Autodesk Inventor part; units mm, degrees
ref_plane "Work Plane1" through (-21.9731, -18.5883, -14.2) normal (0, 0, -1) x (0, 1, 0)
ref_plane "YZ Plane" through (0, 0, 0) normal (1, 0, 0) x (0, 1, 0)
ref_plane "XZ Plane" through (0, 0, 0) normal (0, 1, 0) x (-1, 0, 0)
sketch "Sketch1" plane through (0, 0, 0) normal (0, 0, 1) x (1, 0, 0)
  line L0 (-11, 18.9) -> (-11, 18.25)
  line L1 (-11, 18.25) -> (-20.7, 18.25)
  line L2 (-20.7, 18.25) -> (-20.7, -18.25)
  line L3 (-11, -18.25) -> (-20.7, -18.25)
  line L4 (-11, -18.25) -> (-11, -18.9)
  line L5 (0, -18.9) -> (-11, -18.9)
  line L6 (0, -18.25) -> (0, -18.9)
  line L7 (9.7, -18.25) -> (0, -18.25)
  line L8 (9.7, 18.25) -> (9.7, -18.25)
  line L9 (9.7, 18.25) -> (0, 18.25)
  line L10 (0, 18.9) -> (0, 18.25)
  line L11 (0, 18.9) -> (-11, 18.9)
  circle A0 centre (-5.5, 0) radius 11.5
  circle A1 centre (-5.5, 0) radius 13.5
  point P0 (0, 0)
  dimension "d0" = 2
extrude "Extrusion1" add sketch "Sketch1" along normal blind 4 contours L11 L10 L9 L8 L7 L6 L5 L4 L3 L2 L1 L0
sketch "Sketch2" plane through (0, 0, 4) normal (0, 0, 1) x (1, 0, 0)
  line L0 (-11, 18.9) -> (-11, 18.25)
  line L1 (-11, 18.25) -> (-20.7, 18.25)
  line L2 (-20.7, 18.25) -> (-20.7, -18.25)
  line L3 (-20.7, -18.25) -> (-11, -18.25)
  line L4 (-11, -18.25) -> (-11, -18.9)
  line L5 (-11, -18.9) -> (0, -18.9)
  line L6 (0, -18.9) -> (0, -18.25)
  line L7 (0, -18.25) -> (9.7, -18.25)
  line L8 (9.7, -18.25) -> (9.7, 18.25)
  line L9 (9.7, 18.25) -> (0, 18.25)
  line L10 (0, 18.25) -> (0, 18.9)
  line L11 (0, 18.9) -> (-11, 18.9)
  circle A0 centre (-5.5, 0) radius 13.5
  line L12 (13.7, 22.25) -> (13.7, -22.25)
  line L13 (13.7, -22.25) -> (6, -22.25)
  line L14 (-17, -22.25) -> (-24.7, -22.25)
  line L15 (-24.7, -22.25) -> (-24.7, 22.25)
  line L16 (-24.7, 22.25) -> (-17, 22.25)
  line L17 (6, 22.25) -> (13.7, 22.25)
  line L18 (10.2, 18.75) -> (10.2, -18.75)
  line L19 (10.2, -18.75) -> (0.5, -18.75)
  line L20 (0.5, -18.75) -> (0.5, -19.4)
  line L21 (0.5, -19.4) -> (-11.5, -19.4)
  line L22 (-11.5, -19.4) -> (-11.5, -18.75)
  line L23 (-11.5, -18.75) -> (-21.2, -18.75)
  line L24 (-21.2, -18.75) -> (-21.2, 18.75)
  line L25 (-21.2, 18.75) -> (-11.5, 18.75)
  line L26 (-11.5, 18.75) -> (-11.5, 19.4)
  line L27 (-11.5, 19.4) -> (0.5, 19.4)
  line L28 (0.5, 19.4) -> (0.5, 18.75)
  line L29 (0.5, 18.75) -> (10.2, 18.75)
  line L30 (-17, -22.25) -> (6, -22.25)
  line L31 (6, 22.25) -> (-17, 22.25)
  point P0 (0, 0)
  dimension "d3" = 4
  dimension "d4" = 0.5
ref_plane "Work Plane1" through (-21.9731, -18.5883, -14.2) normal (0, 0, -1) x (0, 1, 0)
extrude "Extrusion2" add sketch "Sketch2" against normal up to surface (18.2 mm away) contours L12 L13 L30 L14 L15 L16 L31 L17
extrude "Extrusion3" add sketch "Sketch2" against normal blind 4 contours L18 L19 L20 L21 L22 L23 L24 L25 L26 L27 L28 L29
sketch "Sketch3" plane through (-24.7, -22.25, 4) normal (-1, 0, 0) x (0, 0, 1)
  line L0 (0, 44.5) -> (-18.2, 44.5) construction
  line L1 (-18.2, 44.5) -> (0, 0) construction
  line L2 (0, 0) -> (-18.2, 0) construction
  line L3 (0, 44.5) -> (0, 0) construction
  line L4 (-18.2, 0) -> (0, 44.5) construction
  line L5 (0, 44.5) -> (-9.1, 22.25) construction
  line L6 (0, 22.25) -> (-18.2, 22.25) construction
  line L7 (-18.2, 3.5) -> (-18.2, 41) construction
  line L8 (-18.2, 22.25) -> (0, 44.5) construction
  line L9 (0, 22.25) -> (-18.2, 44.5) construction
  line L10 (-9.1, 33.375) -> (0, 33.375) construction
  line L11 (0, 33.375) -> (-18.2, 44.5) construction
  line L12 (0, 44.5) -> (-18.2, 33.375) construction
  line L13 (-18.2, 44.5) -> (-18.2, 0) construction
  circle A0 centre (-9.1, 38.9375) radius 1.6
  circle A1 centre (-9.1, 5.5625) radius 1.6
  point P0 (-4, 22.25)
  dimension "d9" = 3.2
extrude "Extrusion4" cut sketch "Sketch3" against normal through all
sketch "Sketch4" plane through (-24.7, 22.25, 4) normal (0, 1, 0) x (1, 0, 0)
  line L0 (0, 0) -> (0, 18.2) construction
  line L1 (38.4, 18.2) -> (0, 0) construction
  line L2 (0, 0) -> (0, 18.2) construction
  line L3 (0, 18.2) -> (38.4, 0) construction
  circle A0 centre (19.2, 9.1) radius 1.6
  point P0 (24.7, 4)
  dimension "d12" = 3.2
extrude "Extrusion5" cut sketch "Sketch4" against normal through all
sketch "Sketch5" plane through (0, 0, 4) normal (0, 0, 1) x (1, 0, 0)
  line L0 (13.7, 22.25) -> (-24.7, 22.25)
  line L1 (13.7, 22.25) -> (-24.7, 22.25)
  line L2 (-24.7, 22.25) -> (-24.7, 32.25)
  line L3 (-24.7, 32.25) -> (13.7, 32.25)
  line L4 (13.7, 32.25) -> (13.7, 22.25)
  line L5 (-24.7, 22.25) -> (-24.7, -22.25)
  line L6 (-24.7, 22.25) -> (-34.7, 22.25)
  line L7 (-34.7, 22.25) -> (-34.7, -22.25)
  line L8 (-34.7, -22.25) -> (-24.7, -22.25)
  line L9 (-24.7, -22.25) -> (-24.7, 22.25)
  line L10 (13.7, 27.25) -> (-24.7, 27.25) construction
  line L11 (-29.7, 22.25) -> (-29.7, -22.25) construction
  circle A0 centre (8.7, 27.25) radius 1.6
  circle A1 centre (-29.7, -17.25) radius 1.6
  circle A2 centre (-29.7, -7.25) radius 1.6
  line L12 (-24.7, 0) -> (-34.7, 0) construction
  circle A3 centre (-29.7, 17.25) radius 1.6
  circle A4 centre (-29.7, 7.25) radius 1.6
  line L13 (-5.5, 22.25) -> (-5.5, 32.25) construction
  circle A5 centre (-1.3, 27.25) radius 1.6652
  circle A6 centre (-19.7, 27.25) radius 1.6
  circle A7 centre (-9.7, 27.25) radius 1.6652
  line L14 (13.7, 22.25) -> (-24.7, 22.25)
  line L15 (-24.7, 22.25) -> (-24.7, -22.25)
  line L16 (-24.7, -22.25) -> (13.7, -22.25)
  line L17 (13.7, -22.25) -> (13.7, 22.25)
  circle A8 centre (-5.5, 0) radius 13.5
  point P0 (0, 0)
  dimension "d15" = 10
  dimension "d16" = 10
  dimension "d17" = 3.2
  dimension "d18" = 5
  dimension "d19" = 3.2
  dimension "d20" = 5
  dimension "d21" = 10
  dimension "d22" = 3.2
  dimension "d23" = 10
extrude "Extrusion6" add sketch "Sketch5" along normal blind 2.5
properties part number "bau_holder"
CAD build for the part. Positions are in the model's coordinates, mm. A direction names the side the tool comes from. Give positions to 0.01 mm unless a question says otherwise; leave off trailing zeros. Loops run counter-clockwise (first coordinate to the right, second up) from the corner with the lowest first, then second, coordinate; pieces in that order, holes last. Notation, with made-up numbers: (81.5, 22.5) -> (87.5, 22.5) arc R20 cw to (87.5, 48.5) -> close; hole circle Ø8 at (13.25, 8). An arc over 180 degrees is marked (long way). Use a Markdown table: item, result.
1. Slice it at C-C (z = 2.5). List the corners of the cut face in (x, y), plus the area to 3 significant figures.
Check result:
| item | result |
|---|---|
| outline | (-24.7, -22.25) -> (13.7, -22.25) -> (13.7, 22.25) -> (-24.7, 22.25) -> close; hole circle Ø27 at (-5.5, 0) |
| area | 1,140 mm^2 |
2. Slice it at B-B (x = -29.7). List the corners of the cut face in (y, z).
Check result:
| item | result |
|---|---|
| outline | (-22.25, 4) -> (-18.85, 4) -> (-18.85, 6.5) -> (-22.25, 6.5) -> close; (-15.65, 4) -> (-8.85, 4) -> (-8.85, 6.5) -> (-15.65, 6.5) -> close; (-5.65, 4) -> (5.65, 4) -> (5.65, 6.5) -> (-5.65, 6.5) -> close; (8.85, 4) -> (15.65, 4) -> (15.65, 6.5) -> (8.85, 6.5) -> close; (18.85, 4) -> (22.25, 4) -> (22.25, 6.5) -> (18.85, 6.5) -> close |
3. Slice it at D-D (y = -6.5). List the corners of the cut face in (x, z), plus the area to 3 significant figures.
Check result:
| item | result |
|---|---|
| outline | (-34.7, 4) -> (-31.11, 4) -> (-31.11, 6.5) -> (-34.7, 6.5) -> close; (-28.29, 4) -> (-24.7, 4) -> (-24.7, -14.2) -> (-21.2, -14.2) -> (-21.2, 0) -> (-17.33, 0) -> (-17.33, 6.5) -> (-28.29, 6.5) -> close; (6.33, 0) -> (10.2, 0) -> (10.2, -14.2) -> (13.7, -14.2) -> (13.7, 6.5) -> (6.33, 6.5) -> close |
| area | 213 mm^2 |
4. Slice it at A-A (y = 27.25). List the corners of the cut face in (x, z).
Check result:
| item | result |
|---|---|
| outline | (-24.7, 4) -> (-21.3, 4) -> (-21.3, 6.5) -> (-24.7, 6.5) -> close; (-18.1, 4) -> (-11.37, 4) -> (-11.37, 6.5) -> (-18.1, 6.5) -> close; (-8.03, 4) -> (-2.97, 4) -> (-2.97, 6.5) -> (-8.03, 6.5) -> close; (0.37, 4) -> (7.1, 4) -> (7.1, 6.5) -> (0.37, 6.5) -> close; (10.3, 4) -> (13.7, 4) -> (13.7, 6.5) -> (10.3, 6.5) -> close |
5. Flat gauge pins, fed straight in: pin 1 (9 mm diameter, centred on y = 2.5, z = -5, fed in from -X); pin 2 (5 mm diameter, centred on x = -28.5, y = 2, fed in from -Z); pin 3 (1.5 mm diameter, centred on x = -18, y = 8.5, fed in from -Z). Where does each tip first touch, or does it go through?
Check result:
| item | result |
|---|---|
| pin 1 | stops at x = -24.7 |
| pin 2 | stops at z = 4 |
| pin 3 | stops at z = 0 |
6. Mould opens along Z. For faces 1 (the flat face through (-6, 32.25, 5)), 2 (the cylindrical face through (-6.68, 20.84, -6.18)), 3 (the flat face through (-6, 27, 4)) say: pulls with the +Z half, pulls with the -Z half, needs draft (parallel to the pull), parting line crosses it, or undercut.
Check result:
| item | result |
|---|---|
| face 1 | needs draft |
| face 2 | undercut |
| face 3 | pulls with the -Z half |
7. Wall check: L1, parallel to Y at x = -29.7, z = 4.8; L2, parallel to X at y = -10, z = -8.25; L3, parallel to Y at x = -22.55, z = -5.1. Give the ranges that are in metal, low to high. Write a range as [from, to].
Check result:
| item | result |
|---|---|
| L1 | y = [-22.25, -18.85], [-15.65, -8.85], [-5.65, 5.65], [8.85, 15.65], [18.85, 22.25] |
| L2 | x = [-24.7, -21.2], [10.2, 13.7] |
| L3 | y = [-22.25, -18.29], [-15.09, 15.09], [18.29, 22.25] |
8. Which spindle directions (+Z, -Z, +X, -X, +Y, -Y) get a long thin tool onto all of the face, cutting with end or side? Do faces 4 (the flat face through (-30, 22.25, 5)), 5 (the flat face through (-6, 22.25, -3)), 6 (the flat face through (-16, 11, 6.5)), 7 (the flat face through (-5, -19.4, -7)). Say none if no direction does.
Check result:
| item | result |
|---|---|
| face 4 | +Z, -Z, -X, +Y |
| face 5 | -Z, +X, -X, +Y |
| face 6 | +Z, +X, -X, +Y, -Y |
| face 7 | -Z |
